```python
from build123d import *

# Parameters (mm, degrees)
EXTRUDE_1_DEPTH     = 40
SKETCH_2_R          = 7.5
SKETCH_2_W          = 12
SKETCH_2_H          = 10
CUT_EXTRUDE_1_DEPTH = 48.843494856
SKETCH_3_W          = 25
SKETCH_3_H          = 7
EXTRUDE_2_DEPTH     = 25
CUT_EXTRUDE_2_REACH = 57.371
SKETCH_4_R          = 6
SKETCH_6_W          = 8
SKETCH_6_H          = 8
CUT_EXTRUDE_3_DEPTH = 45.665422868


with BuildPart() as part:
    # Эскиз1 → Бобышка-Вытянуть1 (new body)
    with BuildSketch(Plane.XY):
        Polygon((-25, 4), (-25, -4), (17, -4), (17, 2), (25, 2), (25, 4), align=None)
    extrude(amount=EXTRUDE_1_DEPTH)

    # Эскиз2 → Вырез-Вытянуть1 (cut, through all)
    with BuildSketch(Plane(origin=(0, 4, 0), x_dir=(1, 0, 0), z_dir=(0, 1, 0))):
        with Locations((-15, 0)):
            Circle(SKETCH_2_R)
        with Locations((-19, -28)):
            Rectangle(SKETCH_2_W, SKETCH_2_H)
    extrude(amount=-CUT_EXTRUDE_1_DEPTH, mode=Mode.SUBTRACT)

    # Эскиз3 → Бобышка-Вытянуть2 (add)
    with BuildSketch(Plane(origin=(0, 4, 0), x_dir=(1, 0, 0), z_dir=(0, 1, 0))):
        with Locations((-0.5, -36.5)):
            Rectangle(SKETCH_3_W, SKETCH_3_H)
        with Locations((-0.5, -19.5)):
            Rectangle(SKETCH_3_W, SKETCH_3_H)
    extrude(amount=EXTRUDE_2_DEPTH)

    # Эскиз4 → Вырез-Вытянуть2 (cut, up to next)
    with BuildSketch(Plane.XY.offset(40), mode=Mode.PRIVATE) as cut_extrude_2_sk1:
        with Locations((-13, 14)):
            Circle(SKETCH_4_R)
    cut_extrude_2_tool1 = extrude(cut_extrude_2_sk1.sketch, amount=-CUT_EXTRUDE_2_REACH, mode=Mode.PRIVATE) & part.part
    add(cut_extrude_2_tool1.solids().sort_by_distance((-13, 14, 40))[0], mode=Mode.SUBTRACT)

    # Эскиз6 → Вырез-Вытянуть3 (cut, through all)
    with BuildSketch(Plane.XY.offset(23)):
        with Locations((-9, 12)):
            Rectangle(SKETCH_6_W, SKETCH_6_H)
    extrude(amount=-CUT_EXTRUDE_3_DEPTH, mode=Mode.SUBTRACT)


solid = part.part
```
The listing builds one solid part. Answer for the finished solid, in the listing's coordinates (mm). A direction names the side the tool comes from. Give positions to 0.01 mm unless a question says otherwise; leave off trailing zeros. Loops run counter-clockwise (first coordinate to the right, second up) from the corner with the lowest first, then second, coordinate; pieces in that order, holes last. Notation, with made-up numbers: M 80.5,57.5 L 93.5,57.5 A17 cw 93.5,85.5 Z; hole C -39,-22 d8. An arc over 180 degrees is marked long. One line per item, written item: value.
1. Find the intervals of material crossed by probe 1 along Z at (x, y) = (-11, 6); probe 2 along Y at (x, z) = (8, 2); probe 3 along X at (y, z) = (26.5, 22), in increasing order.
Found:
probe 1: 16 to 23, 33 to 40
probe 2: -4 to 4
probe 3: -13 to 12
2. For faces 1 (the face through (-19, 0, 33)), 2 (the face through (-13, 6, 20)), 3 (the face through (-9, 16, 20)), determine the directions among +Z, -Z, +X, -X, +Y, -Y from which every point of the face is accessible in a straight line to the end or side of a thin tool.
Found:
face 1: -X, +Y, -Y
face 2: +Z, -Z, -X, +Y
face 3: -Z, -X
3. For a pull along Z with two mould halves and no side action, classify faces 4 (the face through (-7, 14, 37)), 5 (the face through (6, 4, 15)), 6 (the face through (5, 0, 0)) as pulls with the +Z half, pulls with the -Z half, needs draft (parallel to the pull), parting line crosses it, or undercut.
Found:
face 4: needs draft
face 5: undercut
face 6: pulls with the -Z half
4. Section D-D on x = -1 is taken. Determine the outline of the cut face in (y, z).
Found:
outline: M -4,0 L 4,0 L 4,16 L 29,16 L 29,23 L 4,23 L 4,33 L 29,33 L 29,40 L -4,40 Z
5. Each of these flat-tipped pins is pushed along its axis until it touches: P1, Ø8, axis at x = 20, z = 18.5, coming from the +Y side; P2, Ø2, axis at y = 22, z = 19, coming from the -X side; P3, Ø3.5, axis at y = 11, z = 19, coming from the +X side; P4, Ø6.5, axis at x = 19, z = 29.5, coming from the -Y side. Where does it stop, or does it pass through?
Found:
P1: y = 4
P2: x = -13
P3: x = 12
P4: y = -4
6. Section C-C on z = 31 is taken. Determine the outline of the cut face in (x, y).
Found:
outline: M -13,-4 L 17,-4 L 17,2 L 25,2 L 25,4 L -13,4 Z
7. Section B-B on x = -15 is taken. Determine the outline of the cut face in (y, z).
Found:
outline: M -4,7.5 L 4,7.5 L 4,23 L -4,23 Z; M -4,33 L 4,33 L 4,40 L -4,40 Z
8. Section A-A on y = 7 is taken. Determine the outline of the cut face in (x, z).
Found:
outline: M -13,16 L 12,16 L 12,23 L -13,23 Z; M -13,33 L 12,33 L 12,40 L -13,40 Z
